from build123d import *

# Parameters (mm, degrees)
SKETCH1_R           = 105
SKETCH1_R_2         = 1.5
BOSS_EXTRUDE1_DEPTH = 5
SKETCH2_R           = 1.8
CUT_EXTRUDE1_DEPTH  = 2.5
SKETCH2_3_R         = 1.8
CUT_EXTRUDE3_DEPTH  = 149.576579581
CUT_EXTRUDE4_DEPTH  = 149.576579581


with BuildPart() as part:
    # Sketch1 → Boss-Extrude1 (new body)
    with BuildSketch(Plane(origin=(0, 0, 0), x_dir=(1, 0, 0), z_dir=(0, 1, 0))):
        with Locations(Location((0, 0, 0), (0, 0, 270))):
            Circle(SKETCH1_R)
        with Locations(Location((-27.5, 30, 0), (0, 0, 270))):
            Circle(SKETCH1_R_2, mode=Mode.SUBTRACT)
        with Locations(Location((27.5, 30, 0), (0, 0, 90))):
            Circle(SKETCH1_R_2, mode=Mode.SUBTRACT)
        with Locations(Location((27.5, -30, 0), (0, 0, 270))):
            Circle(SKETCH1_R_2, mode=Mode.SUBTRACT)
        with Locations(Location((-27.5, -30, 0), (0, 0, 90))):
            Circle(SKETCH1_R_2, mode=Mode.SUBTRACT)
    extrude(amount=BOSS_EXTRUDE1_DEPTH)

    # Sketch2 → Cut-Extrude1 (cut)
    # profile 1 of 8: a face of its own
    with BuildSketch(Plane(origin=(0, 5, 0), x_dir=(1, 0, 0), z_dir=(0, 1, 0))):
        Polygon((0, -65.762029021), (2.825, -64.13101451), (2.825, -60.86898549), (0, -59.237970979), (-2.825, -60.86898549), (-2.825, -64.13101451), align=None)
        with Locations((0, -62.5)):
            Circle(SKETCH2_R, mode=Mode.SUBTRACT)
    # profile 2 of 8: a face of its own
    with BuildSketch(Plane(origin=(0, 5, 0), x_dir=(1, 0, 0), z_dir=(0, 1, 0))):
        with Locations((0, -62.5)):
            Circle(SKETCH2_R)
    # profile 3 of 8: a face of its own
    with BuildSketch(Plane(origin=(0, 5, 0), x_dir=(1, 0, 0), z_dir=(0, 1, 0))):
        Polygon((-65.762029021, 0), (-64.13101451, -2.825), (-60.86898549, -2.825), (-59.237970979, 0), (-60.86898549, 2.825), (-64.13101451, 2.825), align=None)
        with Locations((-62.5, 0)):
            Circle(SKETCH2_R, mode=Mode.SUBTRACT)
    # profile 4 of 8: a face of its own
    with BuildSketch(Plane(origin=(0, 5, 0), x_dir=(1, 0, 0), z_dir=(0, 1, 0))):
        with Locations((-62.5, 0)):
            Circle(SKETCH2_R)
    # profile 5 of 8: a face of its own
    with BuildSketch(Plane(origin=(0, 5, 0), x_dir=(1, 0, 0), z_dir=(0, 1, 0))):
        Polygon((0, 65.762029021), (-2.825, 64.13101451), (-2.825, 60.86898549), (0, 59.237970979), (2.825, 60.86898549), (2.825, 64.13101451), align=None)
        with Locations((0, 62.5)):
            Circle(SKETCH2_R, mode=Mode.SUBTRACT)
    # profile 6 of 8: a face of its own
    with BuildSketch(Plane(origin=(0, 5, 0), x_dir=(1, 0, 0), z_dir=(0, 1, 0))):
        with Locations((0, 62.5)):
            Circle(SKETCH2_R)
    # profile 7 of 8: a face of its own
    with BuildSketch(Plane(origin=(0, 5, 0), x_dir=(1, 0, 0), z_dir=(0, 1, 0))):
        Polygon((65.762029021, 0), (64.13101451, 2.825), (60.86898549, 2.825), (59.237970979, 0), (60.86898549, -2.825), (64.13101451, -2.825), align=None)
        with Locations((62.5, 0)):
            Circle(SKETCH2_R, mode=Mode.SUBTRACT)
    # profile 8 of 8: a face of its own
    with BuildSketch(Plane(origin=(0, 5, 0), x_dir=(1, 0, 0), z_dir=(0, 1, 0))):
        with Locations((62.5, 0)):
            Circle(SKETCH2_R)
    extrude(amount=-CUT_EXTRUDE1_DEPTH, mode=Mode.SUBTRACT)

    # Sketch2_3 → Cut-Extrude3 (cut, through all)
    with BuildSketch(Plane(origin=(0, 5, 0), x_dir=(1, 0, 0), z_dir=(0, 1, 0))):
        with Locations(Location((0, 62.5, 0), (0, 0, 270))):
            Circle(SKETCH2_3_R)
        with Locations(Location((62.5, 0, 0), (0, 0, 270))):
            Circle(SKETCH2_3_R)
        with Locations(Location((0, -62.5, 0), (0, 0, 270))):
            Circle(SKETCH2_3_R)
        with Locations(Location((-62.5, 0, 0), (0, 0, 270))):
            Circle(SKETCH2_3_R)
    extrude(amount=-CUT_EXTRUDE3_DEPTH, mode=Mode.SUBTRACT)

    # Sketch4 → Cut-Extrude4 (cut, through all)
    with BuildSketch(Plane(origin=(0, 5, 0), x_dir=(1, 0, 0), z_dir=(0, 1, 0))):
        with BuildLine():
            Line((-103, -20.396078054), (-103, 20.396078054))
            ThreePointArc((-103, 20.396078054), (-105, 0), (-103, -20.396078054))
        make_face()
        with BuildLine():
            Line((20.396078054, -103), (-20.396078054, -103))
            ThreePointArc((-20.396078054, -103), (0, -105), (20.396078054, -103))
        make_face()
        with BuildLine():
            ThreePointArc((105, 0), (104.498803821, 10.246950766), (103, 20.396078054))
            Line((103, 20.396078054), (103, -20.396078054))
            ThreePointArc((103, -20.396078054), (104.498803821, -10.246950766), (105, 0))
        make_face()
        with BuildLine():
            ThreePointArc((20.396078054, 103), (0, 105), (-20.396078054, 103))
            Line((-20.396078054, 103), (20.396078054, 103))
        make_face()
    extrude(amount=-CUT_EXTRUDE4_DEPTH, mode=Mode.SUBTRACT)


solid = part.part
Could you check a few things on this model? Use its own coordinates, in mm. A direction names the side the tool comes from. Give positions to 0.01 mm unless a question says otherwise; leave off trailing zeros. Order: outer loops, then holes, each group sorted by start corner. A loop starts at its lowest first (then second) coordinate and runs counter-clockwise, first axis right, second up.
1. Thinking about a two-plate mould opening in Z: for faces 3 (the cylindrical face through (-74.86, 2.46, 73.63)), 4 (the flat face through (0, 3, -103)), 5 (the flat face through (-2, 2.5, 62)), 6 (the flat face through (-63, 2.5, -2)), which applies, +Z half, -Z half, draft (parallel to the pull), parting line (faces both ways), or undercut?
Answers below:
face 3: +Z half
face 4: -Z half
face 5: undercut
face 6: undercut
2. Suppose I cut it at C-C (x = 83). Write out the boundary of the cut face in (y, z), plus the area to 3 significant figures.
Answers below:
outline: (0, -64.31) - (5, -64.31) - (5, 64.31) - (0, 64.31) - close
area: 643 mm2
3. For pin 1 (3 mm diameter, centred on y = 3, z = -47, fed in from +X); pin 2 (2 mm diameter, centred on x = -62.5, y = 3.5, fed in from -Z); pin 3 (3 mm diameter, centred on x = -0.5, z = -63, fed in from +Y), each with a flat end and sliding along its axis, tell me the tip position at first contact or that it passes through.
Answers below:
pin 1: stops at x = 94.63
pin 2: stops at z = -85.1
pin 3: stops at y = 2.5
4. Suppose I cut it at B-B (z = 41). Write out the boundary of the cut face in (x, y).
Answers below:
outline: (-96.66, 0) - (96.66, 0) - (96.66, 5) - (-96.66, 5) - close
5. I need wall thicknesses on L1, parallel to X at y = 1.9, z = -30; L2, parallel to X at y = 3.65, z = -1; L3, parallel to X at y = 1.2, z = -62.5. Which ranges of each line are inside material? Lowest first, please.
Answers below:
L1: x = -100.62 to -29, -26 to 26, 29 to 100.62
L2: x = -103 to -65.18, -59.82 to 59.82, 65.18 to 103
L3: x = -84.37 to -1.8, 1.8 to 84.37
6. Suppose I cut it at A-A (y = 1.1). State how many separate pieces and enclosed holes the cut face has, plus the area to 3 significant figures.
Answers below:
separate pieces: 1
enclosed holes: 8
area: 34,300 mm2
7. Which directions (+Z, -Z, +X, -X, +Y, -Y) give clear straight access to the entire face, cutting with the end or side of a thin tool? Please do faces 1 (the cylindrical face through (74.86, 2.46, -73.63)), 2 (the flat face through (-2, 2.5, -63)).
Answers below:
face 1: -Z, +X, +Y, -Y
face 2: +Y
